from build123d import *

# Parameters (mm, degrees)
PAD_DEPTH    = 5
CHAMFER_SIZE = 1
FILLET_R     = 1


with BuildPart() as part:
    # Sketch → Pad (new body)
    with BuildSketch(Plane.XY):
        with BuildLine():
            ThreePointArc((0, 7.5), (-7.5, 0), (0, -7.5))
            Line((0, -7.5), (15, -7.5))
            ThreePointArc((15, -7.5), (22.5, 0), (15, 7.5))
            Line((0, 7.5), (15, 7.5))
        make_face()
        Polygon((2.309401, 4), (-2.309401, 4), (-4.618802, 0), (-2.309401, -4), (2.309401, -4), (4.618802, 0), align=None, mode=Mode.SUBTRACT)
        Polygon((12.690599, 4), (10.381198, 0), (12.690599, -4), (17.309401, -4), (19.618802, 0), (17.309401, 4), align=None, mode=Mode.SUBTRACT)
    extrude(amount=PAD_DEPTH)

    # Chamfer
    chamfer_edges = [part.edges().sort_by_distance(p)[0] for p in [
        (11.535898, 2, 5),
        (15, 4, 5),
        (18.464102, 2, 5),
        (18.464102, -2, 5),
        (15, -4, 5),
        (11.535898, -2, 5),
        (3.464102, 2, 5),
        (0, 4, 5),
        (-3.464102, 2, 5),
        (-3.464102, -2, 5),
        (0, -4, 5),
        (3.464102, -2, 5),
    ]]
    chamfer(chamfer_edges, length=CHAMFER_SIZE)

    # Fillet
    fillet_edges = [part.edges().sort_by_distance(p)[0] for p in [
        (7.5, -7.5, 0),
    ]]
    fillet(fillet_edges, radius=FILLET_R)


solid = part.part
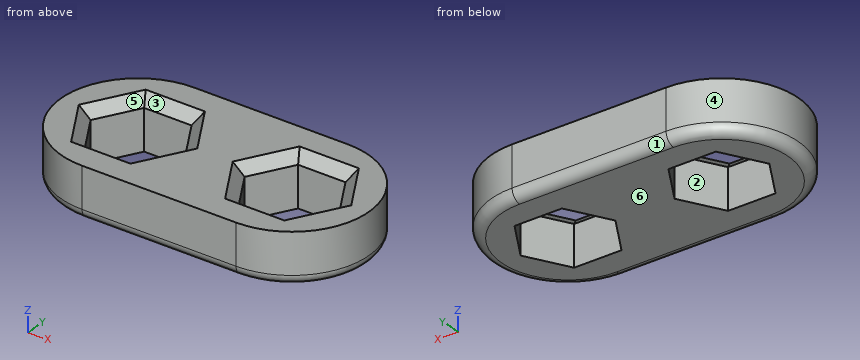
Model file for the job. Use its own axes, mm. Face numbers are marked on the shaded views. A direction names the side the tool comes from. Give positions to 0.01 mm unless a question says otherwise; leave off trailing zeros. Order: outer loops, then holes, each group sorted by start corner. A loop starts at its lowest first (then second) coordinate and runs counter-clockwise, first axis right, second up. Notation, with made-up numbers: (63.25, 8) - (101.25, 8) arc R23 cw to (101.25, 38) - close; hole circle Ø10 at (55, 11). An arc over 180 degrees is marked (long way). Return JSON: item names as keys, results as strings.
1) Cut at A-A, the plane z = 1.65. Give the cut face in (x, y), plus the area to 3 significant figures.
Geometry says:
{"outline": "(0, -7.5) - (15, -7.5) arc R7.5 ccw to (15, 7.5) - (0, 7.5) arc R7.5 ccw to start; hole (-4.62, 0) - (-2.31, -4) - (2.31, -4) - (4.62, 0) - (2.31, 4) - (-2.31, 4) - close; hole (10.38, 0) - (12.69, -4) - (17.31, -4) - (19.62, 0) - (17.31, 4) - (12.69, 4) - close", "area": "291 mm²"}
2) Pull direction Y, two halves, no side cores. Call the marked faces 4, 5 and 6: pulls with the +Y half, pulls with the -Y half, needs draft (parallel to the pull), parting line crosses it, or undercut.
Geometry says:
{"face 4": "parting line crosses it", "face 5": "undercut", "face 6": "needs draft"}
3) Flat gauge pin, fed straight in: P1, Ø2, axis at x = -0.5, z = 2, coming from the +Y side. Where does the tip first touch, or does it go through?
Geometry says:
{"P1": "y = 7.5"}
4) 3-axis set-ups, long thin cutter, end or side, ignore diameter. For the marked faces 1, 2 and 3: which of +Z, -Z, +X, -X, +Y, -Y reach the whole face in a straight line?
Geometry says:
{"face 1": "-Z, +X, -X, +Y", "face 2": "+Z, -Z", "face 3": "+Z"}
5) Cut at C-C, the plane z = 4.65. Give the cut face in (x, y), plus the area to 3 significant figures.
Geometry says:
{"outline": "(0, -7.5) - (15, -7.5) arc R7.5 ccw to (15, 7.5) - (0, 7.5) arc R7.5 ccw to start; hole (-5.37, 0) - (-2.68, -4.65) - (2.68, -4.65) - (5.37, 0) - (2.68, 4.65) - (-2.68, 4.65) - close; hole (9.63, 0) - (12.32, -4.65) - (17.68, -4.65) - (20.37, 0) - (17.68, 4.65) - (12.32, 4.65) - close", "area": "252 mm²"}
6) Probe line 1 (Y direction, x = 2.25, z = 3.95); line 2 (X direction, y = -1.5, z = 2.15); line 3 (X direction, y = -0.5, z = 2). List the from-to ranges inside material, lowest first. Write a range as from..to.
Geometry says:
{"line 1": "-7.5..-4, 4..7.5", "line 2": "-7.35..-3.75, 3.75..11.25, 18.75..22.35", "line 3": "-7.48..-4.33, 4.33..10.67, 19.33..22.48"}
7) Cut at B-B, the plane y = 2.75. Count the separate pieces of the cut face and the enclosed holes in it, plus the area to 3 significant figures.
Geometry says:
{"separate pieces": "3", "enclosed holes": "0", "area": "81.4 mm²"}
